Geometry check sheet. Reference: the model listing, model coordinates, mm. A direction names the side the tool comes from. Round coordinates to 2 decimals unless told otherwise and drop trailing zeros. Order: outer loops, then holes, each group sorted by start corner. A loop starts at its lowest first (then second) coordinate and runs counter-clockwise, first axis right, second up.
(1) Sectioned sample at D-D (x = 5). Record the boundary of the cut face in (y, z), plus the area to 3 significant figures.
(2) Sectioned sample at C-C (y = 0.5). Record the boundary of the cut face in (x, z), plus the area to 3 significant figures.
(3) Sectioned sample at A-A (y = 6). Record the boundary of the cut face in (x, z), plus the area to 3 significant figures.
(4) Sectioned sample at B-B (z = -5). Record the boundary of the cut face in (x, y), plus the area to 3 significant figures.
(5) Material ranges on line 1 along Z through (x, y) = (6.5, 3.75); line 2 along Y through (x, z) = (2.5, -2.25), recorded low to high.
(6) Set-up check for faces 4 (the face through (5, 4, -11.5)), 5 (the face through (9.913, 0.6, -9)): record each of +Z, -Z, +X, -X, +Y, -Y from which the full face is reachable in a straight line by a thin tool's end or side.
(7) Go/stop test with flat-tipped pins: pin 1 (5 mm diameter, centred on x = 3.5, y = 7, fed in from +Z); pin 2 (3 mm diameter, centred on x = 5, z = -7.5, fed in from +Y); pin 3 (4 mm diameter, centred on x = 8, y = 2, fed in from +Z). Record where each tip stops, or that it passes through.
(8) Release check for a two-part mould opening along Y. For faces 1 (the face through (5, 4, -12.5)), 2 (the face through (4.5, 4.3, -12)), 3 (the face through (5, 1, -7)) record: +Y half, -Y half, draft (parallel to the pull), parting line (faces both ways), or undercut.
from build123d import *

# Parameters (mm, degrees)
SKETCH1_W           = 9.91326949
SKETCH1_H           = 11.5
SKETCH1_R           = 1.75
BOSS_EXTRUDE3_DEPTH = 1
SKETCH1_5_W         = 9.91326949
SKETCH1_5_H         = 1
BOSS_EXTRUDE4_DEPTH = 10.5
SKETCH2_R           = 1.75
CUT_EXTRUDE1_DEPTH  = 1


with BuildPart() as part:
    # Sketch1 → Boss-Extrude3 (new body)
    with BuildSketch(Plane(origin=(0, 0, 0), x_dir=(1, 0, 0), z_dir=(0, 1, 0))):
        with Locations((4.956634745, 5.75)):
            Rectangle(SKETCH1_W, SKETCH1_H)
        with Locations(Location((5, 5, 0), (0, 0, 270))):
            Circle(SKETCH1_R, mode=Mode.SUBTRACT)
    extrude(amount=BOSS_EXTRUDE3_DEPTH)

    # Sketch1_5 → Boss-Extrude4 (add)
    with BuildSketch(Plane(origin=(0, 0, 0), x_dir=(1, 0, 0), z_dir=(0, 1, 0))):
        with Locations((4.956634745, 12)):
            Rectangle(SKETCH1_5_W, SKETCH1_5_H)
    extrude(amount=BOSS_EXTRUDE4_DEPTH)

    # Sketch2 → Cut-Extrude1 (cut)
    with BuildSketch(Plane.XY.offset(-11.5)):
        with Locations((4.91326949, 6)):
            Circle(SKETCH2_R)
    extrude(amount=-CUT_EXTRUDE1_DEPTH, mode=Mode.SUBTRACT)


solid = part.part
Answer below:
1. outline: (0, -12.5) - (4.25, -12.5) - (4.25, -11.5) - (1, -11.5) - (1, -6.75) - (0, -6.75) - close; (0, -3.25) - (1, -3.25) - (1, 0) - (0, 0) - close; (7.75, -12.5) - (10.5, -12.5) - (10.5, -11.5) - (7.75, -11.5) - close
1. area: 15.0 mm2
2. outline: (0, -12.5) - (9.91, -12.5) - (9.91, 0) - (0, 0) - close; hole circle Ø3.5 at (5, -5)
2. area: 114 mm2
3. outline: (0, -12.5) - (3.16, -12.5) - (3.16, -11.5) - (0, -11.5) - close; (6.66, -12.5) - (9.91, -12.5) - (9.91, -11.5) - (6.66, -11.5) - close
3. area: 6.41 mm2
4. outline: (0, 0) - (3.25, 0) - (3.25, 1) - (0, 1) - close; (6.75, 0) - (9.91, 0) - (9.91, 1) - (6.75, 1) - close
4. area: 6.41 mm2
5. line 1: z = -12.5 to -11.5
5. line 2: y = 0 to 1
6. face 4: +Z, +X, -X, +Y
6. face 5: +Z, -Z, +X, +Y, -Y
7. pin 1: stops at z = -11.5
7. pin 2: stops at y = 1
7. pin 3: stops at z = 0
8. face 1: draft
8. face 2: undercut
8. face 3: +Y half
